from build123d import *

# Parameters (mm, degrees)
ESQUISSE1_W        = 150
ESQUISSE1_H        = 30
BOSS_EXTRU_1_DEPTH = 5
CONG_1_R           = 6


with BuildPart() as part:
    # Esquisse1 → Boss.-Extru.1 (new body)
    with BuildSketch(Plane.XY):
        Rectangle(ESQUISSE1_W, ESQUISSE1_H)
        Polygon((58.353196257, -6.646803743), (51.706392514, 0), (58.353196257, 6.646803743), (65, 0), align=None, mode=Mode.SUBTRACT)
    extrude(amount=BOSS_EXTRU_1_DEPTH)

    # Congé1
    cong_1_edges = [part.edges().sort_by_distance(p)[0] for p in [
        (75, -15, 2.5),
        (-75, -15, 2.5),
        (-75, 15, 2.5),
        (75, 15, 2.5),
    ]]
    fillet(cong_1_edges, radius=CONG_1_R)


solid = part.part
For this review, take the finished solid that the model builds, in its own axes (mm). A direction names the side the tool comes from. Coordinates: 2 decimals unless noted, no trailing zeros. Write each loop counter-clockwise with the first axis right and the second up, starting at its lowest first coordinate (ties: lowest second). Pieces come first, ordered by that corner, then holes. Notation, with made-up numbers: (44.5, 77.5) -> (99.5, 77.5) arc R19 ccw to (99.5, 114.5) -> close; hole circle Ø10 at (56, 82.25). An arc over 180 degrees is marked (long way). Write each question's results on one line, items separated by ' | '. Start each with the question number.
1) Wall thickness on L1, parallel to X at y = 5.25, z = 3.9; L2, parallel to X at y = 4, z = 3.8; L3, parallel to X at y = 12.75, z = 3.2: over which ranges is each line inside the solid? List them lowest first. Write a range as [from, to].
2) The part is to be moulded in two halves that separate along X. For faces 3 (the face through (-73.289, 13.196, 2.535)), 4 (the face through (73.196, 13.289, 2.535)), 5 (the face through (54.983, 3.277, 2.465)), 6 (the face through (62, 3, 2)), say which applies: +X half, -X half, draft (parallel to the pull), parting line (faces both ways), or undercut.
3) Consider section A-A (z = 1.1). Write out the cut boundary in (x, y).
4) Consider section B-B (y = 3.75). Write out the cut boundary in (x, z).
5) For faces 1 (the face through (75, 0, 2)), 2 (the face through (55.076, -3.37, 2.465)), list the 3-axis set-ups (+Z, -Z, +X, -X, +Y, -Y) from which the entire face can be reached by the end or side of a thin tool; tool diameter is ignored.
6) Consider section C-C (x = 54.5). Write out the cut boundary in (y, z), plus the area to 3 significant figures.
Geometry says:
1) L1: [-75, 56.96], [59.75, 75] | L2: [-75, 55.71], [61, 75] | L3: [-73.68, 73.68]
2) face 3: -X half | face 4: +X half | face 5: undercut | face 6: undercut
3) outline: (-75, -9) arc R6 ccw to (-69, -15) -> (69, -15) arc R6 ccw to (75, -9) -> (75, 9) arc R6 ccw to (69, 15) -> (-69, 15) arc R6 ccw to (-75, 9) -> close; hole (51.71, 0) -> (58.35, -6.65) -> (65, 0) -> (58.35, 6.65) -> close
4) outline: (-75, 0) -> (55.46, 0) -> (55.46, 5) -> (-75, 5) -> close; (61.25, 0) -> (75, 0) -> (75, 5) -> (61.25, 5) -> close
5) face 1: +Z, -Z, +X, +Y, -Y | face 2: +Z, -Z
6) outline: (-15, 0) -> (-2.79, 0) -> (-2.79, 5) -> (-15, 5) -> close; (2.79, 0) -> (15, 0) -> (15, 5) -> (2.79, 5) -> close | area: 122 mm^2
